Design review of the part built by this model. Coordinates are the model's own, in mm. Face numbers are marked on the shaded views. A direction names the side the tool comes from. Round coordinates to 2 decimals unless told otherwise and drop trailing zeros. Order: outer loops, then holes, each group sorted by start corner. A loop starts at its lowest first (then second) coordinate and runs counter-clockwise, first axis right, second up. Notation, with made-up numbers: M 87,-16.75 L 127,-16.75 A38 cw 127,22.25 Z; hole C 62,72.25 d11. An arc over 180 degrees is marked long. Use a Markdown table: item, result. Add a question column.
(1) Machinability: for the marked faces 4, 5, 6, 7 and 8, which of the approach directions +Z, -Z, +X, -X, +Y, -Y give a long, thin tool a straight path to every point of the face, cutting with its end or side? Answer none if there is none.
(2) Take a section at D-D (z = 35.5). Write out the cut boundary in (x, y).
(3) Take a section at B-B (x = -2). Write out the cut boundary in (y, z).
(4) The part is to be moulded in two halves that separate along Y. For the marked faces 1, 2 and 3, say which applies: released by +Y, released by -Y, zero draft, split by the parting line, or undercut.
(5) For pin 1 (12 mm diameter, centred on x = -60.5, y = 12, fed in from -Z); pin 2 (7.5 mm diameter, centred on x = 84.5, y = 4, fed in from -Z); pin 3 (2.5 mm diameter, centred on x = -21.5, y = 6.5, fed in from +Z); pin 4 (7.5 mm diameter, centred on x = -39.5, z = -53, fed in from +Y), all flat-tipped, find the tip position at first contact; note any pin that passes through.
(6) Take a section at C-C (z = 0). Write out the cut boundary in (x, y).
(7) To check wall thickness, follow probe 1 along Z at (x, y) = (52, 18); probe 2 along Y at (x, z) = (10, 0); probe 3 along X at (y, z) = (4, -54.5). State the ranges of each line that lie inside material, in increasing order. Write a range as from..to.
(8) Take a section at A-A (y = 18). Write out the cut boundary in (x, z).
```python
from build123d import *

# Parameters (mm, degrees)
BOSS_EXTRUDE1_DEPTH     = 15
SKETCH2_W               = 200
SKETCH2_H               = 80
BOSS_EXTRUDE2_DEPTH     = 15
BOSS_EXTRUDE3_DEPTH     = 200
CUT_EXTRUDE1_DEPTH      = 214.703065022
CUT_EXTRUDE1_DEPTH_BACK = 214.703065022
SKETCH4_R               = 7


with BuildPart() as part:
    # Sketch1 → Boss-Extrude1 (new body)
    with BuildSketch(Plane(origin=(0, 0, 0), x_dir=(1, 0, 0), z_dir=(0, 1, 0))):
        Polygon((-60, 50), (-57.355095289, 65), (-47.355095289, 65), (-44.710190579, 50), (-40, 50), (-37.355095289, 65), (-27.355095289, 65), (-24.710190579, 50), (-20, 50), (-17.355095289, 65), (-7.355095289, 65), (-4.710190579, 50), (0, 50), (2.644904711, 65), (12.644904711, 65), (15.289809421, 50), (20, 50), (22.644904711, 65), (32.644904711, 65), (35.289809421, 50), (40, 50), (42.644904711, 65), (52.644904711, 65), (55.289809421, 50), (100, 50), (100, -50), (55.289809421, -50), (52.644904711, -65), (42.644904711, -65), (40, -50), (35.289809421, -50), (32.644904711, -65), (22.644904711, -65), (20, -50), (15.289809421, -50), (12.644904711, -65), (2.644904711, -65), (0, -50), (-4.710190579, -50), (-7.355095289, -65), (-17.355095289, -65), (-20, -50), (-24.710190579, -50), (-27.355095289, -65), (-37.355095289, -65), (-40, -50), (-44.710190579, -50), (-47.355095289, -65), (-57.355095289, -65), (-60, -50), (-100, -50), (-100, 50), align=None)
    extrude(amount=BOSS_EXTRUDE1_DEPTH)

    # Sketch2 → Boss-Extrude2 (add)
    with BuildSketch(Plane(origin=(0, 15, 0), x_dir=(1, 0, 0), z_dir=(0, 1, 0))):
        Rectangle(SKETCH2_W, SKETCH2_H)
    extrude(amount=BOSS_EXTRUDE2_DEPTH)

    # Sketch3 → Boss-Extrude3 (add)
    with BuildSketch(Plane.ZY.offset(100)):
        Polygon((25, 30), (29.618802154, 38), (9.618802154, 38), (14.237604307, 30), align=None)
        Polygon((-25, 30), (-14.237604307, 30), (-9.618802154, 38), (-29.618802154, 38), align=None)
    extrude(amount=-BOSS_EXTRUDE3_DEPTH)

    # Sketch4 → Cut-Extrude1 (cut, two sides: drawn at the far end of the back side and taken through both)
    with BuildSketch(Plane.ZY.offset(100).offset(-CUT_EXTRUDE1_DEPTH_BACK)):
        with Locations((0, 18)):
            Circle(SKETCH4_R)
    extrude(amount=CUT_EXTRUDE1_DEPTH + CUT_EXTRUDE1_DEPTH_BACK, mode=Mode.SUBTRACT)


solid = part.part
```
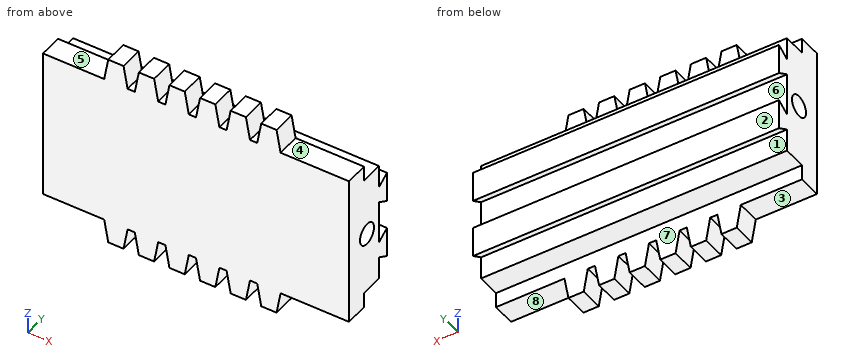
Verdict:
| question | item | result |
|---|---|---|
| 1 | face 4 | +Z, +X, +Y, -Y |
| 1 | face 5 | +Z, -X, +Y, -Y |
| 1 | face 6 | +X, -X |
| 1 | face 7 | -Z, +X, -X, +Y |
| 1 | face 8 | -Z, +X, +Y, -Y |
| 2 | outline | M -100,0 L 100,0 L 100,30 L -100,30 Z |
| 3 | outline | M 0,-50 L 15,-50 L 15,-40 L 30,-40 L 30,-25 L 38,-29.62 L 38,-9.62 L 30,-14.24 L 30,14.24 L 38,9.62 L 38,29.62 L 30,25 L 30,40 L 15,40 L 15,50 L 0,50 Z; hole C 18,0 d14 |
| 4 | face 1 | undercut |
| 4 | face 2 | released by +Y |
| 4 | face 3 | zero draft |
| 5 | pin 1 | stops at z = -65 |
| 5 | pin 2 | stops at z = -50 |
| 5 | pin 3 | stops at z = 50 |
| 5 | pin 4 | stops at y = 15 |
| 6 | outline | M -100,0 L 100,0 L 100,11 L -100,11 Z; M -100,25 L 100,25 L 100,30 L -100,30 Z |
| 7 | probe 1 | z = -40..-7, 7..40 |
| 7 | probe 2 | y = 0..11, 25..30 |
| 7 | probe 3 | x = -59.21..-45.5, -39.21..-25.5, -19.21..-5.5, 0.79..14.5, 20.79..34.5, 40.79..54.5 |
| 8 | outline | M -100,-40 L 100,-40 L 100,-7 L -100,-7 Z; M -100,7 L 100,7 L 100,40 L -100,40 Z |
